from build123d import *

# Parameters (mm, degrees)
F0_R      = 28.575
F1_DEPTH  = 32
F2_DEPTH  = 22
F4_DEPTH  = 95.001
F5_W      = 12
F5_H      = 50
F5_W_2    = 10
F6_DEPTH  = 110
F8_DEPTH  = 10
F9_R      = 11.1
F10_DEPTH = 32.001


with BuildPart() as f1:
    # F0 (on Front) → F1 (new body, symmetric)
    with BuildSketch(Plane.XZ):
        with BuildLine():
            ThreePointArc((35.142567, -41), (49.05965, -22.564368), (54, 0))
            ThreePointArc((54, 0), (49.05965, 22.564368), (35.142567, 41))
            ThreePointArc((35.142567, 41), (-54, 0), (35.142567, -41))
        make_face()
        Circle(F0_R, mode=Mode.SUBTRACT)
    extrude(amount=F1_DEPTH, both=True)

    # F0 (on Front) → F2 (join, symmetric)
    with BuildSketch(Plane.XZ):
        with BuildLine():
            ThreePointArc((35.142567, 41), (49.05965, 22.564368), (54, 0))
            ThreePointArc((54, 0), (49.05965, -22.564368), (35.142567, -41))
            Line((35.142567, -41), (174, -41))
            Line((174, -41), (174, 41))
            Line((174, 41), (35.142567, 41))
        make_face()
    extrude(amount=F2_DEPTH, both=True)

    # F3 (on face) → F4 (cut, through all)
    with BuildSketch(Plane.XY.offset(41)):
        Polygon((174, -10), (162, -22), (174, -22), align=None)
    extrude(amount=-F4_DEPTH, mode=Mode.SUBTRACT)

    # F5 (on face) → F6 (cut)
    with BuildSketch(Plane.YZ.offset(174)):
        with Locations((-16, 0)):
            Rectangle(F5_W, F5_H)
        with Locations((-5, 0)):
            Rectangle(F5_W_2, F5_H)
    extrude(amount=-F6_DEPTH, mode=Mode.SUBTRACT)

    # F7 (on face) → F8 (join)
    with BuildSketch(Plane.XZ.offset(32)):
        with BuildLine():
            Line((-23.675528, 16), (-51.575188, 16))
            ThreePointArc((-51.575188, 16), (-54, 0), (-51.575188, -16))
            Line((-51.575188, -16), (-23.675528, -16))
            ThreePointArc((-23.675528, -16), (-28.575, 0), (-23.675528, 16))
        make_face()
        with BuildLine():
            Line((51.575188, 16), (23.675528, 16))
            ThreePointArc((23.675528, 16), (27.322691, 8.366672), (28.575, 0))
            ThreePointArc((28.575, 0), (27.322691, -8.366672), (23.675528, -16))
            Line((23.675528, -16), (51.575188, -16))
            ThreePointArc((51.575188, -16), (53.390356, -8.091349), (54, 0))
            ThreePointArc((54, 0), (53.390356, 8.091349), (51.575188, 16))
        make_face()
    extrude(amount=F8_DEPTH)

    # F9 (on face) → F10 (cut, through all)
    with BuildSketch(Plane.XZ):
        with Locations((89, 0)):
            Circle(F9_R)
        with Locations((139, 0)):
            Circle(F9_R)
    extrude(amount=-F10_DEPTH, mode=Mode.SUBTRACT)


solid = f1.part
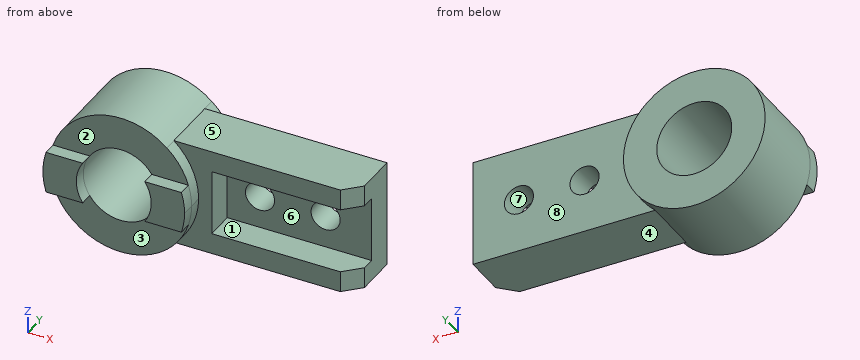
Could you check a few things on this model? Use its own coordinates, in mm. Face numbers are marked on the shaded views. A direction names the side the tool comes from. Round coordinates to 2 decimals unless told otherwise and drop trailing zeros. Write each loop counter-clockwise with the first axis right and the second up, starting at its lowest first coordinate (ties: lowest second). Pieces come first, ordered by that corner, then holes. Notation, with made-up numbers: (26.25, 84) - (49.25, 84) arc R26 cw to (49.25, 103) - close; hole circle Ø11 at (-23, 60). An arc over 180 degrees is marked (long way). Use a Markdown table: item, result.
Q1. For pin 1 (17.5 mm diameter, centred on x = 123, y = -11.5, fed in from +Z); pin 2 (3 mm diameter, centred on x = 38, y = -35.5, fed in from -Z); pin 3 (8 mm diameter, centred on y = -23, z = -16.5, fed in from -X), each with a flat end and sliding along its axis, tell me the tip position at first contact or that it passes through.
Output values:
| item | result |
|---|---|
| pin 1 | z = 41 |
| pin 2 | z = -16 |
| pin 3 | x = -52.53 |
Q2. I want a section at D-D (z = 33). List the corners of the cut face in (x, y) for me, plus the area to 3 significant figures.
Output values:
| item | result |
|---|---|
| outline | (-42.74, -32) - (42.74, -32) - (42.74, -22) - (162, -22) - (174, -10) - (174, 22) - (42.74, 22) - (42.74, 32) - (-42.74, 32) - close |
| area | 11,200 mm2 |
Q3. Thinking about a two-plate mould opening in Z: for the marked faces 5, 6, 7 and 8, which applies, released by +Z, released by -Z, zero draft, split by the parting line, or undercut?
Output values:
| item | result |
|---|---|
| face 5 | released by +Z |
| face 6 | undercut |
| face 7 | undercut |
| face 8 | zero draft |
Q4. I want a section at A-A (x = 0). List the corners of the cut face in (y, z) for me (3 decimals), plus the area to 3 significant figures.
Output values:
| item | result |
|---|---|
| outline | (-32, -54) - (32, -54) - (32, -28.575) - (-32, -28.575) - close; (-32, 28.575) - (32, 28.575) - (32, 54) - (-32, 54) - close |
| area | 3,250 mm2 |
Q5. For the marked faces 1, 2, 3 and 4, which set-ups out of +Z, -Z, +X, -X, +Y, -Y let a thin tool reach every point of the face, with its end or its side?
Output values:
| item | result |
|---|---|
| face 1 | +X, -Y |
| face 2 | +Z, +X, -X, -Y |
| face 3 | -Z, +X, -X, -Y |
| face 4 | -Z, +X, +Y, -Y |
Q6. Please list where these lines run through material, in increasing order: L1, parallel to Z at x = 0, y = -9 (3 decimals); L2, parallel to Z at x = 89, y = 14; L3, parallel to X at y = -6, z = 0 (3 decimals).
Output values:
| item | result |
|---|---|
| L1 | -54 to -28.575, 28.575 to 54 |
| L2 | -41 to -11.1, 11.1 to 41 |
| L3 | -54 to -28.575, 28.575 to 64 |
Q7. I want a section at B-B (z = -4). List the corners of the cut face in (x, y) for me.
Output values:
| item | result |
|---|---|
| outline | (-53.85, -42) - (-28.29, -42) - (-28.29, 32) - (-53.85, 32) - close; (28.29, -42) - (53.85, -42) - (53.85, -22) - (64, -22) - (64, 0) - (78.65, 0) - (78.65, 22) - (53.85, 22) - (53.85, 32) - (28.29, 32) - close; (99.35, 0) - (128.65, 0) - (128.65, 22) - (99.35, 22) - close; (149.35, 0) - (174, 0) - (174, 22) - (149.35, 22) - close |
Q8. I want a section at C-C (x = 75.5). List the corners of the cut face in (y, z) for me, plus the area to 3 significant figures.
Output values:
| item | result |
|---|---|
| outline | (-22, -41) - (22, -41) - (22, 41) - (-22, 41) - (-22, 25) - (0, 25) - (0, -25) - (-22, -25) - close |
| area | 2,510 mm2 |
